Verification items for the finished model (mm, model axes). Face numbers are marked on the shaded views. A direction names the side the tool comes from. Round coordinates to 2 decimals unless told otherwise and drop trailing zeros. Order: outer loops, then holes, each group sorted by start corner. A loop starts at its lowest first (then second) coordinate and runs counter-clockwise, first axis right, second up. Notation, with made-up numbers: M -1,-3.5 L 7,-3.5 A31 ccw 7,23.5 Z; hole C -21,16.5 d9. An arc over 180 degrees is marked long. Return JSON: item names as keys, results as strings. Group by question number.
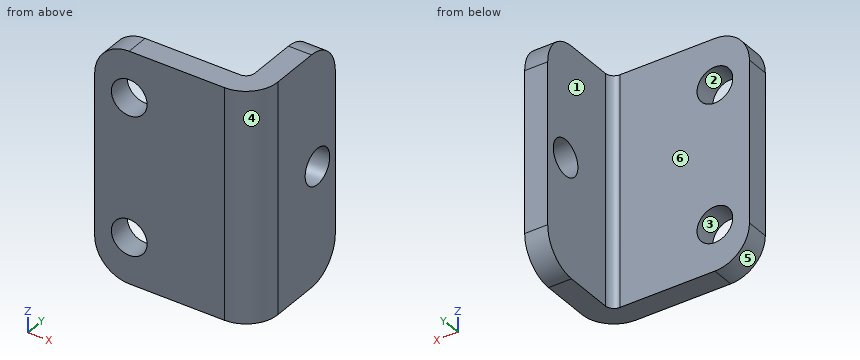
from build123d import *

# Parameters (mm, degrees)
BASE_FLANGE1_DEPTH = 10
FILLET1_R          = 3
SKETCH6_R          = 1.55
CUT_EXTRUDE1_DEPTH = 18.549928775
SKETCH7_R          = 1.55
CUT_EXTRUDE2_DEPTH = 18.549928775


# Sheet-metal steps are written as plain solids
with BuildPart() as part:
    # Sketch1 → Base-Flange1 (new, symmetric)
    with BuildSketch(Plane.XY):
        with BuildLine():
            Line((-12, 0), (-0.75, 0))
            ThreePointArc((-0.75, 0), (-0.219669914, 0.219669914), (0, 0.75))
            Line((0, 0.75), (0, 8))
            Line((0, 8), (2, 8))
            Line((2, 8), (2, 0.75))
            ThreePointArc((2, 0.75), (1.194543648, -1.194543648), (-0.75, -2))
            Line((-0.75, -2), (-12, -2))
            Line((-12, -2), (-12, 0))
        make_face()
    extrude(amount=BASE_FLANGE1_DEPTH, both=True)

    # Fillet1
    fillet1_edges = [part.edges().sort_by_distance(p)[0] for p in [
        (-12, -1, 10),
        (1, 8, 10),
        (-12, -1, -10),
        (1, 8, -10),
    ]]
    fillet(fillet1_edges, radius=FILLET1_R)

    # Sketch6 → Cut-Extrude1 (cut, through all)
    with BuildSketch(Plane(origin=(0, 0, 0), x_dir=(1, 0, 0), z_dir=(0, 1, 0))):
        with Locations(Location((-9, 6, 0), (0, 0, 270))):
            Circle(SKETCH6_R)
        with Locations(Location((-9, -6, 0), (0, 0, 90))):
            Circle(SKETCH6_R)
    extrude(amount=-CUT_EXTRUDE1_DEPTH, mode=Mode.SUBTRACT)

    # Sketch7 → Cut-Extrude2 (cut, through all)
    with BuildSketch(Plane.ZY):
        with Locations((0, 5.75)):
            Circle(SKETCH7_R)
    extrude(amount=-CUT_EXTRUDE2_DEPTH, mode=Mode.SUBTRACT)


solid = part.part
1. Thickness scan on line 1 along X through (y, z) = (3, 8); line 2 along Y through (x, z) = (-8, -7.5); line 3 along X through (y, z) = (-0.55, 6). Record the ranges inside material, lowest first. Write a range as from..to.
2. Cross-section at D-D (y = 5.5). Enter the section's corners in (x, z).
3. Cross-section at A-A (z = 6). Enter the section's corners in (x, y).
4. Draft check along X on the marked faces 3, 4, 5 and 6. Enter one of: +X half, -X half, draft (parallel to the pull), parting line (faces both ways), or undercut.
5. Access from +Z, -Z, +X, -X, +Y, -Y to the whole of each face (thin tool, end or side, straight path). Record for the marked faces 1 and 2.
6. Go/stop test with flat-tipped pins: pin 1 (3 mm diameter, centred on y = 5, z = 0, fed in from -X); pin 2 (1 mm diameter, centred on x = -2.5, z = 0, fed in from +Y). Record where each tip stops, or that it passes through.
7. Cross-section at C-C (z = -2). Enter the section's corners in (x, y).
8. Cross-section at B-B (y = 7). Enter the section's corners in (x, z), plus the area to 3 significant figures.
Computed:
{
 "1": {"line 1": "x = 0..2", "line 2": "y = -2..0", "line 3": "x = -12..-10.55, -7.45..1.67"},
 "2": {"outline": "M 0,-9.96 L 2,-9.96 L 2,-1.53 L 0,-1.53 Z; M 0,1.53 L 2,1.53 L 2,9.96 L 0,9.96 Z"},
 "3": {"outline": "M -12,-2 L -10.55,-2 L -10.55,0 L -12,0 Z; M -7.45,-2 L -0.75,-2 A2.75 ccw 2,0.75 L 2,8 L 0,8 L 0,0.75 A0.75 cw -0.75,0 L -7.45,0 Z"},
 "4": {"face 3": "undercut", "face 4": "+X half", "face 5": "-X half", "face 6": "draft"},
 "5": {"face 1": "+Z, -Z, -X, +Y", "face 2": "+Y, -Y"},
 "6": {"pin 1": "stops at x = 0", "pin 2": "stops at y = 0"},
 "7": {"outline": "M -12,-2 L -0.75,-2 A2.75 ccw 2,0.75 L 2,8 L 0,8 L 0,0.75 A0.75 cw -0.75,0 L -12,0 Z"},
 "8": {"outline": "M 0,-9.24 L 2,-9.24 L 2,-0.92 L 0,-0.92 Z; M 0,0.92 L 2,0.92 L 2,9.24 L 0,9.24 Z", "area": "33.3 mm²"}
}
